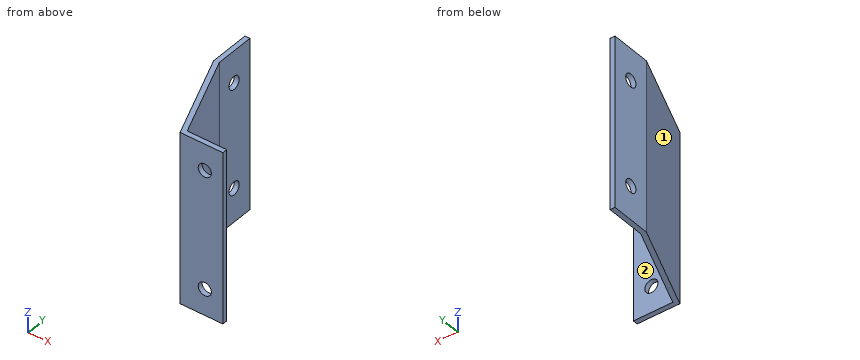
```python
from build123d import *

# Parameters (mm, degrees)
EXTRUDE_THIN1_DEPTH = 165.1
SKETCH2_R           = 6.35
CUT_EXTRUDE1_DEPTH  = 5.7625
SKETCH3_R           = 6.35
CUT_EXTRUDE2_DEPTH  = 5.7625


with BuildPart() as part:
    # Sketch1 → Extrude-Thin1 (new body)
    with BuildSketch(Plane.XY):
        Polygon((0, 120.65), (0, 82.55), (32.995567884, 0), (71.095567884, 0), (71.095567884, -4.7625), (29.770312185, -4.7625), (-4.7625, 81.633456448), (-4.7625, 120.65), align=None)
    extrude(amount=EXTRUDE_THIN1_DEPTH)

    # Sketch2 → Cut-Extrude1 (cut, through all)
    with BuildSketch(Plane(origin=(0, 0, 0), x_dir=(0, 0, -1), z_dir=(1, 0, 0))):
        with Locations((-134.204880657, 100.94227704)):
            Circle(SKETCH2_R)
        with Locations((-32.604880657, 100.94227704)):
            Circle(SKETCH2_R)
    extrude(amount=-CUT_EXTRUDE1_DEPTH, mode=Mode.SUBTRACT)

    # Sketch3 → Cut-Extrude2 (cut, through all)
    with BuildSketch(Plane(origin=(0, 0, 0), x_dir=(1, 0, 0), z_dir=(0, 1, 0))):
        with Locations((53.633067884, -25.4)):
            Circle(SKETCH3_R)
        with Locations((53.633067884, -139.7)):
            Circle(SKETCH3_R)
    extrude(amount=-CUT_EXTRUDE2_DEPTH, mode=Mode.SUBTRACT)


solid = part.part
```
Verification items for the finished model (mm, model axes). Face numbers are marked on the shaded views. A direction names the side the tool comes from. Coordinates: 2 decimals unless noted, no trailing zeros. Loops run counter-clockwise (first coordinate to the right, second up) from the corner with the lowest first, then second, coordinate; pieces in that order, holes last. Notation, with made-up numbers: (-35.5, 29) -> (12.5, 29) arc R26 ccw to (12.5, 64) -> close; hole circle Ø8 at (59.5, 44.25). An arc over 180 degrees is marked (long way). Put each result on its own line as item: value.
1. Tool access check on the marked faces 1 and 2. Record the directions out of +Z, -Z, +X, -X, +Y, -Y that give a thin tool (end or side, any length) a straight path to the whole face; none if there is none.
Result set:
face 1: +Z, -Z, -X, -Y
face 2: +Z, -Z, +X, +Y
2. Section check C-C, the plane y = 60. Record the boundary of the cut face in (x, z).
Result set:
outline: (3.88, 0) -> (9.01, 0) -> (9.01, 165.1) -> (3.88, 165.1) -> close
3. Gauge pin test, flat ends, axial feed: P1, Ø19, axis at x = 51, z = 116.5, coming from the +Y side; P2, Ø1, axis at y = 20.5, z = 49, coming from the +X side. Record the tip position at first contact, or that the pin passes through.
Result set:
P1: stops at y = 0
P2: stops at x = 25
4. Section check B-B, the plane x = 40.5. Record the boundary of the cut face in (y, z).
Result set:
outline: (-4.76, 0) -> (0, 0) -> (0, 165.1) -> (-4.76, 165.1) -> close
5. Thickness scan on line 1 (Y direction, x = 37.5, z = 48); line 2 (X direction, y = -2, z = 25.4). Record the ranges inside material, lowest first.
Result set:
line 1: y = -4.76 to 0
line 2: x = 28.67 to 47.28, 59.98 to 71.1
6. Section check A-A, the plane z = 59. Record the boundary of the cut face in (x, y), then the cut area to 3 significant figures.
Result set:
outline: (-4.76, 81.63) -> (29.77, -4.76) -> (71.1, -4.76) -> (71.1, 0) -> (33, 0) -> (0, 82.55) -> (0, 120.65) -> (-4.76, 120.65) -> close
area: 806 mm^2
